from build123d import *

# Parameters (mm, degrees)
SKETCH1_R           = 8
BOSS_EXTRUDE2_DEPTH = 12
SKETCH3_R           = 8.742551749
BOSS_EXTRUDE3_DEPTH = 12
SKETCH4_R           = 8
BOSS_EXTRUDE4_DEPTH = 12
SKETCH5_R           = 8
BOSS_EXTRUDE5_DEPTH = 12


with BuildPart() as part:
    # Sketch1 → Boss-Extrude2 (new body)
    with BuildSketch(Plane(origin=(0, 0, 0), x_dir=(1, 0, 0), z_dir=(0, 1, 0))):
        with BuildLine():
            Line((-64.715447154, 17.804878049), (15.284552846, 17.804878049))
            ThreePointArc((15.284552846, 17.804878049), (35.284552846, -2.195121951), (15.284552846, -22.195121951))
            Line((15.284552846, -22.195121951), (-64.715447154, -22.195121951))
            Line((-64.715447154, -22.195121951), (-64.715447154, 17.804878049))
        make_face()
        with Locations((15.284552846, -2.195121951)):
            Circle(SKETCH1_R, mode=Mode.SUBTRACT)
    extrude(amount=BOSS_EXTRUDE2_DEPTH)

    # Sketch3 → Boss-Extrude3 (add)
    with BuildSketch(Plane.ZY.offset(64.715447154)):
        with BuildLine():
            ThreePointArc((22.195121951, 34), (2.195121951, 54), (-17.804878049, 34))
            Line((-17.804878049, 34), (-17.804878049, 12))
            Line((-17.804878049, 12), (22.195121951, 12))
            Line((22.195121951, 12), (22.195121951, 34))
        make_face()
        with Locations((2.195121951, 34)):
            Circle(SKETCH3_R, mode=Mode.SUBTRACT)
    extrude(amount=-BOSS_EXTRUDE3_DEPTH)

    # Sketch4 → Boss-Extrude4 (add)
    with BuildSketch(Plane(origin=(0, 0, -17.804878049), x_dir=(-1, 0, 0), z_dir=(0, 0, -1))):
        with BuildLine():
            Line((64.715447154, 0), (64.715447154, -34))
            ThreePointArc((64.715447154, -34), (44.715447154, -54), (24.715447154, -34))
            Line((24.715447154, -34), (24.715447154, 0))
            Line((24.715447154, 0), (64.715447154, 0))
        make_face()
        with Locations((44.715447154, -34)):
            Circle(SKETCH4_R, mode=Mode.SUBTRACT)
    extrude(amount=-BOSS_EXTRUDE4_DEPTH)

    # Sketch5 → Boss-Extrude5 (add)
    with BuildSketch(Plane.XY.offset(22.195121951)):
        with BuildLine():
            Line((-64.715447154, 0), (-64.715447154, -34))
            ThreePointArc((-64.715447154, -34), (-44.715447154, -54), (-24.715447154, -34))
            Line((-24.715447154, -34), (-24.715447154, 0))
            Line((-24.715447154, 0), (-64.715447154, 0))
        make_face()
        with Locations((-44.715447154, -34)):
            Circle(SKETCH5_R, mode=Mode.SUBTRACT)
    extrude(amount=-BOSS_EXTRUDE5_DEPTH)


solid = part.part
Model file for the job. Use its own axes, mm. A direction names the side the tool comes from. Round coordinates to 2 decimals unless told otherwise and drop trailing zeros. Order: outer loops, then holes, each group sorted by start corner. A loop starts at its lowest first (then second) coordinate and runs counter-clockwise, first axis right, second up. Notation, with made-up numbers: M 12.25,16 L 32.25,16 A26 ccw 32.25,52 Z; hole C -9.75,5.25 d10. An arc over 180 degrees is marked long. Write each question's results on one line, items separated by ' | '. Start each with the question number.
(1) Saw through at C-C, the plane x = -16. Give the cut face in (y, z).
(2) Two-plate mould, pull along Z, no slides. Class faces 1 (the face through (35.28, 5.92, 1.76)), 2 (the face through (-3, 0, 2)), 3 (the face through (-8, 12, 2)): pulls with the +Z half, pulls with the -Z half, needs draft (parallel to the pull), parting line crosses it, or undercut.
(3) Which spindle directions (+Z, -Z, +X, -X, +Y, -Y) get a long thin tool onto all of the face, cutting with end or side? Do faces 4 (the face through (-52.715, 24, 2)), 5 (the face through (-52.346, -31.597, -11.889)), 6 (the face through (-24.715, -17, 16)), 7 (the face through (-64.715, 11, 2)), 8 (the face through (-45, -21, 10.195)). Say none if no direction does.
(4) Probe probe 1 along Z at (x, y) = (-57, -1); probe 2 along Y at (x, z) = (31, -5.5); probe 3 along X at (y, z) = (17.5, -2). List the from-to ranges inside material, lowest first. Write a range as from..to.
(5) Saw through at D-D, the plane y = 14.5. Give the cut face in (x, z).
(6) Drop flat-ended pins along their axis: pin 1 (13 mm diameter, centred on x = -44.72, y = -34, fed in from -Z); pin 2 (9.5 mm diameter, centred on y = -23, z = 18, fed in from +X); pin 3 (20 mm diameter, centred on x = -13.5, z = 7, fed in from +Y); pin 4 (6 mm diameter, centred on y = 21, z = -11, fed in from +X). Give the stop position or say it passes through.
(7) Saw through at B-B, the plane z = -11. Give the cut face in (x, y), then the cut area to 3 significant figures.
(8) Saw through at A-A, the plane y = -27.5. Give the cut face in (x, z), then the cut area to 3 significant figures.
Established:
1) outline: M 0,-17.8 L 12,-17.8 L 12,22.2 L 0,22.2 Z
2) face 1: parting line crosses it | face 2: undercut | face 3: needs draft
3) face 4: +Z, -Z, +X, +Y | face 5: +Z, -Z | face 6: +Z, -Z, +X, -Y | face 7: +Z, -Z, -X, +Y, -Y | face 8: +X, -X, -Y
4) probe 1: z = -17.8..-5.8, 10.2..22.2 | probe 2: y = 0..12 | probe 3: x = -64.72..-52.72
5) outline: M -64.72,-17.8 L -52.72,-17.8 L -52.72,22.2 L -64.72,22.2 Z
6) pin 1: passes through | pin 2: stops at x = -24.72 | pin 3: stops at y = 12 | pin 4: stops at x = -52.72
7) outline: M -64.72,-34 A20 ccw -24.72,-34 L -24.72,0 L 30.31,0 L 30.31,12 L -52.72,12 L -52.72,49.03 L -64.72,49.03 Z; hole C -44.72,-34 d16 | area: 3,370 mm^2
8) outline: M -64.72,-17.8 L -49.38,-17.8 L -49.38,-5.8 L -64.72,-5.8 Z; M -64.72,10.2 L -49.38,10.2 L -49.38,22.2 L -64.72,22.2 Z; M -40.05,-17.8 L -24.72,-17.8 L -24.72,-5.8 L -40.05,-5.8 Z; M -40.05,10.2 L -24.72,10.2 L -24.72,22.2 L -40.05,22.2 Z | area: 736 mm^2
